CAD build for the part. Positions are in the model's coordinates, mm. Coordinates: 2 decimals unless noted, no trailing zeros. Loops run counter-clockwise (first coordinate to the right, second up) from the corner with the lowest first, then second, coordinate; pieces in that order, holes last. Notation, with made-up numbers: (88, -18.75) -> (143, -18.75) arc R31 cw to (143, 11.25) -> close; hole circle Ø8 at (-25, 4.5). An arc over 180 degrees is marked (long way). Return JSON: item names as keys, results as strings. Group by question number.
(1) Flat gauge pins, fed straight in: pin 1 Ø12 at (y, z) = (0, 0) entering from +X; pin 2 Ø3 at (x, z) = (-115, 10) entering from +Y; pin 3 Ø2 at (x, z) = (129, 10.5) entering from -Y; pin 4 Ø12 at (x, z) = (153, -12) entering from -Y. Where does each tip first touch, or does it go through?
(2) Saw through at B-B on z = -17. Write the cut outline in (x, y), then the cut area to 3 significant figures.
(3) Probe L1, parallel to X at y = -6, z = 20.5; L2, parallel to Z at x = -59.5, y = 0; L3, parallel to X at y = -5, z = 9. List the from-to ranges inside material, lowest first.
(4) Mould opens along Y. For faces 1 (the face through (300, 11, 0)), 2 (the face through (269.99, 7.19, 13.33)) say: pulls with the +Y half, pulls with the -Y half, needs draft (parallel to the pull), parting line crosses it, or undercut.
(5) Saw through at A-A on x = 144. Write the cut outline in (y, z).
```python
from build123d import *

# Parameters (mm, degrees)
F1_DEPTH = 300
F3_R     = 11
F4_DEPTH = 20
F6_R     = 10
F7_DEPTH = 20


with BuildPart() as f1:
    # F0 (on Right) → F1 (new body, symmetric)
    with BuildSketch(Plane.YZ):
        with BuildLine():
            Line((5, 8.6602540378), (12.5, 21.6506350946))
            ThreePointArc((12.5, 21.6506350946), (0, 25), (-12.5, 21.6506350946))
            Line((-12.5, 21.6506350946), (-5, 8.6602540378))
            ThreePointArc((-5, 8.6602540378), (0, 10), (5, 8.6602540378))
        make_face()
        with BuildLine():
            ThreePointArc((-12.5, 21.6506350946), (-12.5, -21.6506350946), (25, 0))
            ThreePointArc((25, 0), (21.6506350946, 12.5), (12.5, 21.6506350946))
            Line((12.5, 21.6506350946), (5, 8.6602540378))
            ThreePointArc((5, 8.6602540378), (8.6602540378, 5), (10, 0))
            ThreePointArc((10, 0), (-5, -8.6602540378), (-5, 8.6602540378))
            Line((-5, 8.6602540378), (-12.5, 21.6506350946))
        make_face()
    extrude(amount=F1_DEPTH, both=True)

    # F3 (on face) → F4 (cut)
    with BuildSketch(Plane(origin=(0, -12.5, 21.6506350946), x_dir=(1, 0, 0), z_dir=(0, 0.5, -0.8660254038))):
        with BuildLine():
            ThreePointArc((206, 0), (195, 11), (184, 0))
            ThreePointArc((184, 0), (195, -11), (206, 0))
        make_face()
        with Locations((-195, 0)):
            Circle(F3_R)
    extrude(amount=F4_DEPTH, mode=Mode.SUBTRACT)

    # F6 (on face) → F7 (cut)
    with BuildSketch(Plane(origin=(0, 12.5, 21.6506350946), x_dir=(1, 0, 0), z_dir=(0, 0.5, 0.8660254038))):
        with BuildLine():
            ThreePointArc((270, 0), (260, 10), (250, 0))
            ThreePointArc((250, 0), (260, -10), (270, 0))
        make_face()
        with Locations((-260, 0)):
            Circle(F6_R)
    extrude(amount=-F7_DEPTH, mode=Mode.SUBTRACT)


solid = f1.part
```
Geometry results:
{
 "1": {"pin 1": "through", "pin 2": "y = 23.51", "pin 3": "y = -23.12", "pin 4": "y = -24.27"},
 "2": {"outline": "(-300, -18.33) -> (300, -18.33) -> (300, 18.33) -> (-300, 18.33) -> close", "area": "22,000 mm²"},
 "3": {"L1": "-300 to -204.77, -185.23 to 185.23, 204.77 to 300", "L2": "-25 to -10, 10 to 25", "L3": "-300 to -264.69, -255.31 to -206, -184 to 184, 206 to 255.31, 264.69 to 300"},
 "4": {"face 1": "needs draft", "face 2": "undercut"},
 "5": {"outline": "circle Ø50 at (0, 0); hole circle Ø20 at (0, 0)"}
}
